from build123d import *

# Parameters (mm, degrees)
BOSS_EXTRUDE1_DEPTH  = 70
BOSS_EXTRUDE2_DEPTH  = 10
FILLET1_R            = 5
FILLET1_OF_MIRROR1_R = 5


with BuildPart() as part:
    # Sketch1 → Boss-Extrude1 (new body)
    with BuildSketch(Plane(origin=(0, 0, 0), x_dir=(1, 0, 0), z_dir=(0, 1, 0))):
        with BuildLine():
            Line((-61.500129939, 0), (25.499870061, 0))
            Line((25.499870061, 0), (57.174837058, 81.028985343))
            Line((57.174837058, 81.028985343), (38.547484106, 88.310586952))
            Line((38.547484106, 88.310586952), (18.556100358, 37.169837828))
            ThreePointArc((18.556100358, 37.169837828), (8.633917242, 24.701856819), (-6.590826128, 20))
            Line((-6.590826128, 20), (-61.500129939, 20))
            Line((-61.500129939, 20), (-61.500129939, 0))
        make_face()
    extrude(amount=BOSS_EXTRUDE1_DEPTH)

    # Sketch2 → Boss-Extrude2 (add)
    with BuildSketch(Plane(origin=(0, 70, 0), x_dir=(1, 0, 0), z_dir=(0, 1, 0))):
        with BuildLine():
            Line((-52.712841503, 15.588653402), (-64.56499654, -24.411346598))
            Line((-64.56499654, -24.411346598), (-54.23346703, -24.411346598))
            Line((-54.23346703, -24.411346598), (-44.613683261, 4.315907023))
            ThreePointArc((-44.613683261, 4.315907023), (-17.295669473, 1.924485185), (10.065785793, 3.753020511))
            Line((10.065785793, 3.753020511), (14.418892199, -24.411346598))
            Line((14.418892199, -24.411346598), (25.43500346, -24.411346598))
            Line((25.43500346, -24.411346598), (18.121502556, 15.588653402))
            ThreePointArc((18.121502556, 15.588653402), (-17.295669473, 11.924485184), (-52.712841503, 15.588653402))
        make_face()
    boss_extrude2 = extrude(amount=BOSS_EXTRUDE2_DEPTH)

    # Fillet1
    fillet1_edges = [part.edges().sort_by_distance(p)[0] for p in [
        (18.121502556, 75, -15.588653402),
    ]]
    fillet(fillet1_edges, radius=FILLET1_R)

    # Mirror1: Boss-Extrude2 across plane
    add(boss_extrude2.mirror(Plane.ZX.offset(35)))

    # Fillet1 of Mirror1
    fillet1_of_mirror1_edges = [part.edges().sort_by_distance(p)[0] for p in [
        (18.121502556, -5, -15.588653402),
    ]]
    fillet(fillet1_of_mirror1_edges, radius=FILLET1_OF_MIRROR1_R)


solid = part.part
Geometry: final body of the model. Coordinates: model frame, mm. A direction names the side the tool comes from. Coordinates: 2 decimals unless noted, no trailing zeros. Order: outer loops, then holes, each group sorted by start corner. A loop starts at its lowest first (then second) coordinate and runs counter-clockwise, first axis right, second up. Notation, with made-up numbers: (67, 10.5) - (114, 10.5) arc R23 cw to (114, 28.5) - close; hole circle Ø9 at (-14, -17). An arc over 180 degrees is marked (long way). Use one line per item in the form item = value.
1) Section B-B (y = 36). Return loops of the section in (x, z).
Solutions:
outline = (-61.5, -20) - (-6.59, -20) arc R27 cw to (18.56, -37.17) - (38.55, -88.31) - (57.17, -81.03) - (25.5, 0) - (-61.5, 0) - close
2) Section A-A (z = 8.5). Return loops of the section in (x, y), then the cut area to 3 significant figures.
Solutions:
outline = (-59.85, -10) - (-48.91, -10) - (-48.91, 0) - (-59.85, 0) - close; (-59.85, 70) - (-48.91, 70) - (-48.91, 80) - (-59.85, 80) - close; (11.96, -10) - (22.53, -10) - (22.53, 0) - (11.96, 0) - close; (11.96, 70) - (22.53, 70) - (22.53, 80) - (11.96, 80) - close
area = 430 mm^2
3) Ray query, L1, parallel to Z at x = -7.5, y = 28; L2, parallel to Y at x = 16, z = -23; L3, parallel to X at y = 33, z = -76.5. Return the intervals inside material, ascending.
Solutions:
L1 = -20 to 0
L2 = 0 to 70
L3 = 33.93 to 55.4
4) Pin query (flat end, axial travel): pin 1 (16.5 mm diameter, centred on x = -36.5, y = 29, fed in from -Z); pin 2 (2 mm diameter, centred on x = 12.5, y = 6, fed in from -Z); pin 3 (1 mm diameter, centred on x = -16, z = -22, fed in from +Y); pin 4 (6 mm diameter, centred on x = 3.5, y = 45, fed in from +Z). Return the tip coordinate at first contact, or that it passes through.
Solutions:
pin_1 = -20
pin_2 = -28.96
pin_3 = through
pin_4 = 0
5) Set-up query: faces 4 (the face through (-18, 70, -1)), 5 (the face through (-58.556, -4.93, 4.131)), 6 (the face through (-55, 0, 12)), 7 (the face through (-17.68, -4.93, -1.93)), 8 (the face through (-19.323, -4.93, -11.936)). Return all of +Z, -Z, +X, -X, +Y, -Y with unobstructed straight access to the full face (end or side cutting, diameter ignored); none if empty.
Solutions:
face_4 = +Z, +Y
face_5 = -Z, -X, -Y
face_6 = +Z, +X, -X
face_7 = +Z, -Y
face_8 = -Z, -Y
6) Section D-D (y = -3). Return loops of the section in (x, z) (3 decimals).
Solutions:
outline = (-64.565, 24.411) - (-52.713, -15.589) arc R173 cw to (13.23, -14.639) arc R5 ccw to (19.031, -10.617) - (25.435, 24.411) - (14.419, 24.411) - (10.066, -3.753) arc R178.19 ccw to (-44.614, -4.316) - (-54.233, 24.411) - close
7) Section C-C (x = -28.5). Return loops of the section in (y, z), then the cut area to 3 significant figures.
Solutions:
outline = (-10, -12.29) - (0, -12.29) - (0, -20) - (70, -20) - (70, -12.29) - (80, -12.29) - (80, -2.39) - (70, -2.39) - (70, 0) - (0, 0) - (0, -2.39) - (-10, -2.39) - close
area = 1,600 mm^2
8) Mould query, pull axis Y, two halves, no side actions, for faces 1 (the face through (47.99, 34.51, -84.62)), 2 (the face through (-18, 0, -1)), 3 (the face through (-19, 35, 0)). Classes: +Y half, -Y half, draft (parallel to the pull), parting line (faces both ways), or undercut.
Solutions:
face_1 = draft
face_2 = -Y half
face_3 = undercut
